```python
from build123d import *

# Parameters (mm, degrees)
SKETCH1_W           = 104
SKETCH1_H           = 115
BOSS_EXTRUDE1_DEPTH = 104
CUT_EXTRUDE1_DEPTH  = 187.70029459
CUT_EXTRUDE2_DEPTH  = 187.70029459
SKETCH4_R           = 25
CUT_EXTRUDE3_DEPTH  = 187.70029459
SKETCH5_R           = 40
CUT_EXTRUDE4_DEPTH  = 10
CUT_EXTRUDE5_START  = -10
SKETCH6_R           = 40
CUT_EXTRUDE5_DEPTH  = 10
FILLET1_R           = 15
SKETCH8_W           = 104
SKETCH8_H           = 104
SKETCH8_W_2         = 98
SKETCH8_H_2         = 98
BOSS_EXTRUDE2_DEPTH = 10
FILLET2_R           = 5
CUT_EXTRUDE6_DEPTH  = 10
SKETCH12_W          = 52
SKETCH12_H          = 52
CUT_EXTRUDE8_DEPTH  = 187.70029459
CUT_EXTRUDE9_DEPTH  = 194.020724276
SKETCH15_W          = 52.000105155
SKETCH15_H          = 10
CUT_EXTRUDE12_DEPTH = 194.020497647


with BuildPart() as part:
    # Sketch1 → Boss-Extrude1 (new body)
    with BuildSketch(Plane.XY):
        with Locations((52, 57.5)):
            Rectangle(SKETCH1_W, SKETCH1_H)
    extrude(amount=BOSS_EXTRUDE1_DEPTH)

    # Sketch2 → Cut-Extrude1 (cut, through all)
    with BuildSketch(Plane(origin=(104, 0, 0), x_dir=(0, 0, -1), z_dir=(1, 0, 0))):
        Polygon((-104, 115), (-79.592698068, 57.5), (-104, 0), align=None)
        Polygon((0, 115), (-24.407301932, 57.5), (0, 0), align=None)
    extrude(amount=-CUT_EXTRUDE1_DEPTH, mode=Mode.SUBTRACT)

    # Sketch3 → Cut-Extrude2 (cut, through all)
    with BuildSketch(Plane.XY):
        Polygon((0, 115), (24.407301932, 57.5), (0, 0), align=None)
        Polygon((104, 115), (79.592698068, 57.5), (104, 0), align=None)
    extrude(amount=CUT_EXTRUDE2_DEPTH, mode=Mode.SUBTRACT)

    # Sketch4 → Cut-Extrude3 (cut, through all)
    with BuildSketch(Plane(origin=(0, 115, 0), x_dir=(1, 0, 0), z_dir=(0, 1, 0))):
        with Locations(Location((52, -52, 0), (0, 0, 270))):
            Circle(SKETCH4_R)
    extrude(amount=-CUT_EXTRUDE3_DEPTH, mode=Mode.SUBTRACT)

    # Sketch5 → Cut-Extrude4 (cut)
    with BuildSketch(Plane(origin=(0, 115, 0), x_dir=(1, 0, 0), z_dir=(0, 1, 0))):
        with Locations(Location((52, -52, 0), (0, 0, 270))):
            Circle(SKETCH5_R)
    extrude(amount=-CUT_EXTRUDE4_DEPTH, mode=Mode.SUBTRACT)

    # Sketch6 → Cut-Extrude5 (cut)
    with BuildSketch(Plane.XZ.offset(CUT_EXTRUDE5_START)):
        with Locations(Location((52, 52, 0), (0, 0, 90))):
            Circle(SKETCH6_R)
    extrude(amount=CUT_EXTRUDE5_DEPTH, mode=Mode.SUBTRACT)

    # Fillet1
    fillet1_edges = [part.edges().sort_by_distance(p)[0] for p in [
        (52, 57.5, 79.592698068),
        (52, 57.5, 24.407301932),
        (24.407301932, 57.5, 52),
        (79.592698068, 57.5, 52),
    ]]
    fillet(fillet1_edges, radius=FILLET1_R)

    # Sketch8 → Boss-Extrude2 (add)
    with BuildSketch(Plane(origin=(0, 115, 0), x_dir=(1, 0, 0), z_dir=(0, 1, 0))):
        with Locations((52, -52)):
            Rectangle(SKETCH8_W, SKETCH8_H)
        with Locations((52, -52)):
            Rectangle(SKETCH8_W_2, SKETCH8_H_2, mode=Mode.SUBTRACT)
    extrude(amount=BOSS_EXTRUDE2_DEPTH)

    # Fillet2
    fillet2_edges = [part.edges().sort_by_distance(p)[0] for p in [
        (52, 115, 104),
        (52, 115, 0),
        (0, 115, 52),
        (104, 115, 52),
    ]]
    fillet(fillet2_edges, radius=FILLET2_R)

    # Sketch11 → Cut-Extrude6 (cut)
    with BuildSketch(Plane(origin=(0, 115, 0), x_dir=(1, 0, 0), z_dir=(0, 1, 0))):
        with BuildLine():
            Line((97.40784106, -10.935563022), (86.801239342, -21.54216474))
            ThreePointArc((86.801239342, -21.54216474), (82.558598655, -21.54216474), (82.558598655, -17.299524053))
            Line((82.558598655, -17.299524053), (93.165200373, -6.692922335))
            ThreePointArc((93.165200373, -6.692922335), (97.40784106, -6.692922335), (97.40784106, -10.935563022))
        make_face()
        with BuildLine():
            Line((11.514167897, -7.27152721), (22.120769615, -17.878128928))
            ThreePointArc((22.120769615, -17.878128928), (22.120769615, -22.120769615), (17.878128928, -22.120769615))
            Line((17.878128928, -22.120769615), (7.27152721, -11.514167897))
            ThreePointArc((7.27152721, -11.514167897), (7.27152721, -7.27152721), (11.514167897, -7.27152721))
        make_face()
        with BuildLine():
            Line((93.743805248, -96.829236185), (83.13720353, -86.222634468))
            ThreePointArc((83.13720353, -86.222634468), (83.13720353, -81.97999378), (87.379844217, -81.97999378))
            Line((87.379844217, -81.97999378), (97.986445935, -92.586595498))
            ThreePointArc((97.986445935, -92.586595498), (97.986445935, -96.829236185), (93.743805248, -96.829236185))
        make_face()
        with BuildLine():
            Line((7.850132085, -93.165200373), (18.456733803, -82.558598655))
            ThreePointArc((18.456733803, -82.558598655), (22.69937449, -82.558598655), (22.69937449, -86.801239342))
            Line((22.69937449, -86.801239342), (12.092772772, -97.40784106))
            ThreePointArc((12.092772772, -97.40784106), (7.850132085, -97.40784106), (7.850132085, -93.165200373))
        make_face()
    extrude(amount=-CUT_EXTRUDE6_DEPTH, mode=Mode.SUBTRACT)

    # Sketch12 → Cut-Extrude8 (cut, through all)
    with BuildSketch(Plane(origin=(0, 115, 0), x_dir=(1, 0, 0), z_dir=(0, 1, 0))):
        with Locations((78, -78)):
            Rectangle(SKETCH12_W, SKETCH12_H)
    extrude(amount=-CUT_EXTRUDE8_DEPTH, mode=Mode.SUBTRACT)

    # Sketch13 → Cut-Extrude9 (cut, through all)
    with BuildSketch(Plane(origin=(0, 125, 0), x_dir=(1, 0, 0), z_dir=(0, 1, 0))):
        Polygon((101, -52), (104, -52), (104, -104), (52, -103.895424297), (52, -101), (101, -101), align=None)
    extrude(amount=-CUT_EXTRUDE9_DEPTH, mode=Mode.SUBTRACT)

    # Sketch15 → Cut-Extrude12 (cut, through all)
    with BuildSketch(Plane(origin=(-0.208729944, 0, 103.790428823), x_dir=(-0.9999979778024204, 0, -0.002011067147068195), z_dir=(0.002011067147068195, 0, -0.9999979778024204))):
        with Locations((-78.208888098, 120)):
            Rectangle(SKETCH15_W, SKETCH15_H)
    extrude(amount=-CUT_EXTRUDE12_DEPTH, mode=Mode.SUBTRACT)


solid = part.part
```
Model file for the job. Use its own axes, mm. A direction names the side the tool comes from. Give positions to 0.01 mm unless a question says otherwise; leave off trailing zeros. Loops run counter-clockwise (first coordinate to the right, second up) from the corner with the lowest first, then second, coordinate; pieces in that order, holes last. Notation, with made-up numbers: (-5.75, 64.5) - (28.25, 64.5) arc R27 ccw to (28.25, 90.5) - close; hole circle Ø10 at (53, -25.5). An arc over 180 degrees is marked (long way). One line per item, written item: value. Start each with the question number.
1. Pull direction Z, two halves, no side cores. Call faces 5 (the flat face through (32.294, 89.067, 92.992)), 6 (the flat face through (34.78, 105, 33.66)), 7 (the flat face through (27, 120, 101)), 8 (the flat face through (104, 120, 26)): pulls with the +Z half, pulls with the -Z half, needs draft (parallel to the pull), parting line crosses it, or undercut.
2. Slice it at B-B (y = 14). List the corners of the cut face in (x, z).
3. Probe L1, parallel to Y at x = 7, z = 85.5; L2, parallel to Z at x = 33, y = 91; L3, parallel to Z at x = 37, y = 12. List the from-to ranges inside material, lowest first. Write a range as from..to.
4. Slice it at A-A (x = 95.5). List the corners of the cut face in (y, z).
5. Pin check, flat tips, straight feed: pin 1 (21.5 mm diameter, centred on x = 87.5, y = 62.5, fed in from +Z); pin 2 (12 mm diameter, centred on x = 15, y = 33.5, fed in from -Z); pin 3 (8.5 mm diameter, centred on x = 93, z = 16, fed in from +Y). Stop position of each tip, or through.
6. Which spindle directions (+Z, -Z, +X, -X, +Y, -Y) get a long thin tool onto all of the face, cutting with end or side? Do faces 1 (the flat face through (11.008, 89.067, 51.278)), 2 (the cylindrical face through (34.915, 58.165, 33.749)), 3 (the cylindrical face through (7.225, 110.07, 7.319)), 4 (the flat face through (52, 63.4, 81.7)). Say none if no direction does.
Solution:
1. face 5: pulls with the +Z half
1. face 6: undercut
1. face 7: undercut
1. face 8: needs draft
2. outline: (5.94, 5.94) - (98.06, 5.94) - (98.06, 52) - (77, 52) arc R25 cw (long way) to (52, 77) - (52, 98.06) - (5.94, 98.06) - close
3. L1: y = 0..16.49, 98.51..115
3. L2: z = 10.19..35.75, 68.25..93.81
3. L3: z = 5.09..32, 72..98.91
4. outline: (0, 0) - (20.02, 8.5) - (20.02, 52) - (0, 52) - close; (94.98, 8.5) - (114.06, 0.4) arc R5 ccw to (116.02, 0) - (125, 0) - (125, 3) - (115, 3) - (115, 5.82) - (105, 5.82) - (105, 12.84) - (115, 12.84) - (115, 52) - (94.98, 52) - close
5. pin 1: stops at z = 52
5. pin 2: stops at z = 11.67
5. pin 3: stops at y = 115
6. face 1: +Z, -Z, -X
6. face 2: +Y, -Y
6. face 3: +Y
6. face 4: +Z, +X, +Y, -Y
